```python
from build123d import *

# Parameters (mm, degrees)
F0_W           = 76.2
F0_H           = 25.4
F1_DEPTH       = 50.8
F3_D           = 12.7
F3_CBORE_D     = 19.05
F3_CBORE_DEPTH = 6.35
F4_W           = 19.05
F4_H           = 6.35
F5_DEPTH       = 9.525


with BuildPart() as f1:
    # F0 (on Front) → F1 (new body)
    with BuildSketch(Plane.XZ):
        with Locations((38.1, 12.7)):
            Rectangle(F0_W, F0_H)
    extrude(amount=F1_DEPTH)

    # F3 (through all)
    with Locations(Plane.XY.offset(25.4)):
        with Locations((25.4, -25.4), (50.8, -25.4)):
            CounterBoreHole(F3_D / 2, F3_CBORE_D / 2, F3_CBORE_DEPTH)

    # F4 (on face) → F5 (cut)
    with BuildSketch(Plane.XY.offset(25.4)):
        with Locations((38.1, -7.9375)):
            Rectangle(F4_W, F4_H)
    extrude(amount=-F5_DEPTH, mode=Mode.SUBTRACT)


solid = f1.part
```
Model file for the job. Use its own axes, mm. A direction names the side the tool comes from. Give positions to 0.01 mm unless a question says otherwise; leave off trailing zeros. Order: outer loops, then holes, each group sorted by start corner. A loop starts at its lowest first (then second) coordinate and runs counter-clockwise, first axis right, second up.
1) Saw through at B-B, the plane y = -25.4. Write the cut outline in (x, z) (3 decimals), then the cut area to 3 significant figures.
2) Mould opens along Y. For faces 3 (the flat face through (0, -25, 13)), 4 (the cylindrical face through (22.47, -31.034, 9.392)), 5 (the flat face through (38, 0, 13)), 6 (the flat face through (38, -50.8, 13)) say: +Y half, -Y half, draft (parallel to the pull), parting line (faces both ways), or undercut.
3) Wall check: probe 1 along Y at (x, z) = (44, 21); probe 2 along X at (y, z) = (-29, 21.25); probe 3 along X at (y, z) = (-22.5, 11). Give the ranges that are in metal, low to high.
4) Pin check, flat tips, straight feed: pin 1 (1.9 mm diameter, centred on x = 35, y = -8, fed in from +Z) (3 decimals); pin 2 (11.5 mm diameter, centred on x = 50.8, y = -25.4, fed in from -Z). Stop position of each tip, or through.
5) 3-axis set-ups, long thin cutter, end or side, ignore diameter. For faces 1 (the cylindrical face through (44.934, -27.832, 9.392)), 2 (the flat face through (53, -32, 19.05)): which of +Z, -Z, +X, -X, +Y, -Y reach the whole face in a straight line?
6) Saw through at C-C, the plane z = 22. Count the separate pieces of the cut face and the enclosed holes in it, then the cut area to 3 significant figures.
7) Saw through at A-A, the plane x = 25.4. Write the cut outline in (y, z) (3 decimals).
8) Saw through at D-D, the plane z = 3.5. Write the cut outline in (x, y), then the cut area to 3 significant figures.
Computed:
1. outline: (0, 0) - (19.05, 0) - (19.05, 19.05) - (15.875, 19.05) - (15.875, 25.4) - (0, 25.4) - close; (31.75, 0) - (44.45, 0) - (44.45, 19.05) - (41.275, 19.05) - (41.275, 25.4) - (34.925, 25.4) - (34.925, 19.05) - (31.75, 19.05) - close; (57.15, 0) - (76.2, 0) - (76.2, 25.4) - (60.325, 25.4) - (60.325, 19.05) - (57.15, 19.05) - close
1. area: 1,210 mm2
2. face 3: draft
2. face 4: undercut
2. face 5: +Y half
2. face 6: -Y half
3. probe 1: y = -50.8 to -32.07, -18.73 to -11.11, -4.76 to 0
3. probe 2: x = 0 to 16.58, 34.22 to 41.98, 59.62 to 76.2
3. probe 3: x = 0 to 19.75, 31.05 to 45.15, 56.45 to 76.2
4. pin 1: stops at z = 15.875
4. pin 2: passes through
5. face 1: +Z, -Z
5. face 2: +Z
6. separate pieces: 1
6. enclosed holes: 3
6. area: 3,180 mm2
7. outline: (-50.8, 0) - (-31.75, 0) - (-31.75, 19.05) - (-34.925, 19.05) - (-34.925, 25.4) - (-50.8, 25.4) - close; (-19.05, 0) - (0, 0) - (0, 25.4) - (-15.875, 25.4) - (-15.875, 19.05) - (-19.05, 19.05) - close
8. outline: (0, -50.8) - (76.2, -50.8) - (76.2, 0) - (0, 0) - close; hole circle Ø12.7 at (25.4, -25.4); hole circle Ø12.7 at (50.8, -25.4)
8. area: 3,620 mm2
